Verification items for the finished model (mm, model axes). A direction names the side the tool comes from. Coordinates: 2 decimals unless noted, no trailing zeros. Write each loop counter-clockwise with the first axis right and the second up, starting at its lowest first coordinate (ties: lowest second). Pieces come first, ordered by that corner, then holes. Notation, with made-up numbers: M 11,47 L 43,47 A32 cw 43,75 Z; hole C 25,77.5 d10. An arc over 180 degrees is marked long. Answer in a Markdown table with one row per item.
from build123d import *

# Parameters (mm, degrees)
SKETCH2_W                             = 100
SKETCH2_H                             = 100
BOSS_EXTRUDE2_DEPTH                   = 5
TAP_DRILL_FOR_M2X0_4_TAP1_D           = 2
TAP_DRILL_FOR_M2X0_4_TAP1_CSINK_D     = 4.2
TAP_DRILL_FOR_M2X0_4_TAP1_CSINK_ANGLE = 90
TAP_DRILL_FOR_M2X0_4_TAP2_D           = 2
TAP_DRILL_FOR_M2X0_4_TAP2_CSINK_D     = 4.2
TAP_DRILL_FOR_M2X0_4_TAP2_CSINK_ANGLE = 90
CIRPATTERN1_COUNT                     = 4


with BuildPart() as part:
    # Sketch2 → Boss-Extrude2 (new body)
    with BuildSketch(Plane(origin=(0, 0, 0), x_dir=(1, 0, 0), z_dir=(0, 1, 0))):
        with Locations((50, 50)):
            Rectangle(SKETCH2_W, SKETCH2_H)
        with BuildLine():
            Line((23.330847354, 81.669152646), (49.292893219, 55.707106781))
            ThreePointArc((49.292893219, 55.707106781), (50, 55.414213562), (50.707106781, 55.707106781))
            Line((50.707106781, 55.707106781), (76.669152646, 81.669152646))
            ThreePointArc((76.669152646, 81.669152646), (76.96054722, 82.430986431), (76.587637332, 83.156410257))
            ThreePointArc((76.587637332, 83.156410257), (50, 92.5), (23.412362668, 83.156410257))
            ThreePointArc((23.412362668, 83.156410257), (23.03945278, 82.430986431), (23.330847354, 81.669152646))
        make_face(mode=Mode.SUBTRACT)
        with BuildLine():
            Line((81.669152646, 76.669152646), (55.707106781, 50.707106781))
            ThreePointArc((55.707106781, 50.707106781), (55.414213562, 50), (55.707106781, 49.292893219))
            Line((55.707106781, 49.292893219), (81.669152646, 23.330847354))
            ThreePointArc((81.669152646, 23.330847354), (82.430986431, 23.03945278), (83.156410257, 23.412362668))
            ThreePointArc((83.156410257, 23.412362668), (92.5, 50), (83.156410257, 76.587637332))
            ThreePointArc((83.156410257, 76.587637332), (82.430986431, 76.96054722), (81.669152646, 76.669152646))
        make_face(mode=Mode.SUBTRACT)
        with BuildLine():
            Line((76.669152646, 18.330847354), (50.707106781, 44.292893219))
            ThreePointArc((50.707106781, 44.292893219), (50, 44.585786438), (49.292893219, 44.292893219))
            Line((49.292893219, 44.292893219), (23.330847354, 18.330847354))
            ThreePointArc((23.330847354, 18.330847354), (23.03945278, 17.569013569), (23.412362668, 16.843589743))
            ThreePointArc((23.412362668, 16.843589743), (50, 7.5), (76.587637332, 16.843589743))
            ThreePointArc((76.587637332, 16.843589743), (76.96054722, 17.569013569), (76.669152646, 18.330847354))
        make_face(mode=Mode.SUBTRACT)
        with BuildLine():
            Line((18.330847354, 23.330847354), (44.292893219, 49.292893219))
            ThreePointArc((44.292893219, 49.292893219), (44.585786438, 50), (44.292893219, 50.707106781))
            Line((44.292893219, 50.707106781), (18.330847354, 76.669152646))
            ThreePointArc((18.330847354, 76.669152646), (17.569013569, 76.96054722), (16.843589743, 76.587637332))
            ThreePointArc((16.843589743, 76.587637332), (7.5, 50), (16.843589743, 23.412362668))
            ThreePointArc((16.843589743, 23.412362668), (17.569013569, 23.03945278), (18.330847354, 23.330847354))
        make_face(mode=Mode.SUBTRACT)
    extrude(amount=BOSS_EXTRUDE2_DEPTH)

    # Tap Drill for M2x0.4 Tap1 (through all)
    with Locations(Plane(origin=(9, 5, -9), x_dir=(0, 0, 1), z_dir=(0, 1, 0))):
        with Locations((0, 0), (-82, 0), (-82, 82), (0, 82)):
            CounterSinkHole(TAP_DRILL_FOR_M2X0_4_TAP1_D / 2, TAP_DRILL_FOR_M2X0_4_TAP1_CSINK_D / 2, counter_sink_angle=TAP_DRILL_FOR_M2X0_4_TAP1_CSINK_ANGLE)

    # Tap Drill for M2x0.4 Tap2 (through all)
    with Locations(Plane(origin=(2.5, 5, -7.25), x_dir=(0, 0, 1), z_dir=(0, 1, 0))):
        with Locations((0, 0), (4.75, 4.75)):
            tap_drill_for_m2x0_4_tap2 = CounterSinkHole(TAP_DRILL_FOR_M2X0_4_TAP2_D / 2, TAP_DRILL_FOR_M2X0_4_TAP2_CSINK_D / 2, counter_sink_angle=TAP_DRILL_FOR_M2X0_4_TAP2_CSINK_ANGLE)

    # CirPattern1: Tap Drill for M2x0.4 Tap2 ×4 about axis
    cirpattern1_axis = Axis((50, 0, -50), (0, 1, 0))
    for i in range(1, CIRPATTERN1_COUNT):
        add(tap_drill_for_m2x0_4_tap2.rotate(cirpattern1_axis, i * 360 / CIRPATTERN1_COUNT), mode=Mode.SUBTRACT)


solid = part.part
1) Sectioned sample at A-A (x = 25). Record the cut outline in (y, z).
Response values:
| item | result |
|---|---|
| outline | M 0,-100 L 5,-100 L 5,-84.37 L 0,-84.37 Z; M 0,-80 L 5,-80 L 5,-70 L 0,-70 Z; M 0,-30 L 5,-30 L 5,-20 L 0,-20 Z; M 0,-15.63 L 5,-15.63 L 5,0 L 0,0 Z |
2) Thickness scan on L1, parallel to Z at x = 2.5, y = 2.1; L2, parallel to X at y = 2.55, z = -52; L3, parallel to Z at x = 73, y = 4.6. Record the ranges inside material, lowest first. Write a range as [from, to].
Response values:
| item | result |
|---|---|
| L1 | z = [-100, -93.75], [-91.75, -8.25], [-6.25, 0] |
| L2 | x = [0, 7.55], [43, 57], [92.45, 100] |
| L3 | z = [-100, -85.74], [-78, -68], [-32, -22], [-14.26, 0] |
3) Sectioned sample at C-C (y = 2.9). Give the number of separate pieces and of enclosed holes in the cut face, then the cut area to 3 significant figures.
Response values:
| item | result |
|---|---|
| separate pieces | 1 |
| enclosed holes | 16 |
| area | 5,440 mm² |
4) Depth check by flat-ended pin: pin 1 (2 mm diameter, centred on x = 34.5, y = 4, fed in from +Z); pin 2 (3 mm diameter, centred on x = 9, z = -91, fed in from +Y); pin 3 (2.5 mm diameter, centred on x = 2.5, z = -92.75, fed in from +Y). Enter the tip coordinate at first touch or a pass-through.
Response values:
| item | result |
|---|---|
| pin 1 | stops at z = 0 |
| pin 2 | stops at y = 4.4 |
| pin 3 | stops at y = 4.15 |
5) Release check for a two-part mould opening along Z. For faces 1 (the face through (64, 2, -69)), 2 (the face through (49, 2, 0)), 3 (the face through (49.6, 2.5, -7.5)), 4 (the face through (49, 0, -51)) record: +Z half, -Z half, draft (parallel to the pull), parting line (faces both ways), or undercut.
Response values:
| item | result |
|---|---|
| face 1 | undercut |
| face 2 | +Z half |
| face 3 | undercut |
| face 4 | draft |
6) Sectioned sample at B-B (z = -42.5). Record the cut outline in (x, y).
Response values:
| item | result |
|---|---|
| outline | M 0,0 L 8.17,0 L 8.17,5 L 0,5 Z; M 37.5,0 L 47.5,0 L 47.5,5 L 37.5,5 Z; M 52.5,0 L 62.5,0 L 62.5,5 L 52.5,5 Z; M 91.83,0 L 100,0 L 100,5 L 91.83,5 Z |
7) Tool access check on faces 5 (the face through (0, 2, -49)), 6 (the face through (36, 2, -31)). Record the directions out of +Z, -Z, +X, -X, +Y, -Y that give a thin tool (end or side, any length) a straight path to the whole face; none if there is none.
Response values:
| item | result |
|---|---|
| face 5 | +Z, -Z, -X, +Y, -Y |
| face 6 | +Y, -Y |
